from build123d import *

# Parameters (mm, degrees)
CROQUIS1_R              = 1.5
SALIENTE_EXTRUIR1_DEPTH = 3


with BuildPart() as part:
    # Croquis1 → Saliente-Extruir1 (new body)
    with BuildSketch(Plane(origin=(0, 0, 0), x_dir=(1, 0, 0), z_dir=(0, 1, 0))):
        with BuildLine():
            Line((-27.161614769, -3.105), (-9.331998714, -3.105))
            ThreePointArc((-9.331998714, -3.105), (2.40938914, -9.535306444), (9.686839463, 1.700695802))
            Line((9.686839463, 1.700695802), (11.574510255, 2.02597122))
            ThreePointArc((11.574510255, 2.02597122), (13.368530359, 5.198598559), (9.902464329, 6.325744796))
            Line((9.902464329, 6.325744796), (8.227399936, 5.249463408))
            ThreePointArc((8.227399936, 5.249463408), (7.196926129, 5.010869422), (6.248965214, 5.480095872))
            ThreePointArc((6.248965214, 5.480095872), (5.907504818, 6.481199341), (6.278579258, 7.471707855))
            Line((6.278579258, 7.471707855), (7.564320065, 8.991935775))
            ThreePointArc((7.564320065, 8.991935775), (6.899293653, 12.575483213), (3.519617395, 11.210983026))
            Line((3.519617395, 11.210983026), (2.928263966, 9.309793011))
            ThreePointArc((2.928263966, 9.309793011), (2.29224049, 8.464643619), (1.264447351, 8.214754404))
            ThreePointArc((1.264447351, 8.214754404), (0.359376606, 8.762157641), (0.006949519, 9.759453236))
            Line((0.006949519, 9.759453236), (0.014700448, 11.750473647))
            ThreePointArc((0.014700448, 11.750473647), (-2.798199231, 14.068159511), (-4.510097634, 10.850477702))
            Line((-4.510097634, 10.850477702), (-3.741039257, 9.013966998))
            ThreePointArc((-3.741039257, 9.013966998), (-3.685009949, 7.957716993), (-4.31171948, 7.105638053))
            ThreePointArc((-4.31171948, 7.105638053), (-5.356907913, 6.943205), (-6.267931977, 7.480641985))
            Line((-6.267931977, 7.480641985), (-7.541797671, 9.010834307))
            ThreePointArc((-7.541797671, 9.010834307), (-11.186383596, 8.978187623), (-10.429487856, 5.412913271))
            Line((-10.429487856, 5.412913271), (-8.659868635, 4.500405648))
            ThreePointArc((-8.659868635, 4.500405648), (-8.038781185, 3.922072963), (-7.809412295, 3.105))
            Line((-7.809412295, 3.105), (-27.161614769, 3.105))
            ThreePointArc((-27.161614769, 3.105), (-30.266614769, 0), (-27.161614769, -3.105))
        make_face()
        with Locations(Location((0, 0, 0), (0, 0, 270))):
            Circle(CROQUIS1_R, mode=Mode.SUBTRACT)
        with Locations(Location((-27.161614769, 0, 0), (0, 0, 270))):
            Circle(CROQUIS1_R, mode=Mode.SUBTRACT)
    extrude(amount=SALIENTE_EXTRUIR1_DEPTH)


solid = part.part
CAD build for the part. Positions are in the model's coordinates, mm. A direction names the side the tool comes from. Give positions to 0.01 mm unless a question says otherwise; leave off trailing zeros. Order: outer loops, then holes, each group sorted by start corner. A loop starts at its lowest first (then second) coordinate and runs counter-clockwise, first axis right, second up. Notation, with made-up numbers: (29, 3) - (40, 3) arc R19 cw to (40, 21) - close; hole circle Ø3 at (-8.75, 22). An arc over 180 degrees is marked (long way). Answer in a Markdown table with one row per item.
1. Flat gauge pins, fed straight in: pin 1 (1 mm diameter, centred on y = 0.5, z = 4.5, fed in from +X); pin 2 (0.9 mm diameter, centred on x = -22.5, y = 1.5, fed in from +Z) (3 decimals). Where does each tip first touch, or does it go through?
Data:
| item | result |
|---|---|
| pin 1 | stops at x = 8.98 |
| pin 2 | stops at z = 3.105 |
2. Saw through at D-D, the plane z = 5.5. Give the cut face in (x, y).
Data:
| item | result |
|---|---|
| outline | (-8.15, 0) - (8.15, 0) - (8.15, 3) - (-8.15, 3) - close |
3. Tool access for faces 1 (the flat face through (-17, 1, -3.105)), 2 (the flat face through (-4.131, 1.479, -9.945)), 3 (the flat face through (-6.9, 1.48, -8.24)), 4 (the flat face through (6.91, 1.48, -8.22)): list every direction of +Z, -Z, +X, -X, +Y, -Y with a clear straight run to the whole face (end or side of a thin tool).
Data:
| item | result |
|---|---|
| face 1 | -X, +Y, -Y |
| face 2 | +Y, -Y |
| face 3 | -Z, +Y, -Y |
| face 4 | +X, +Y, -Y |
4. Pull direction Z, two halves, no side cores. Call faces 5 (the flat face through (3.228, 1.479, -10.274)), 6 (the cylindrical face through (-8.045, 1.479, -3.932)), 7 (the flat face through (-4, 3, -2)), 8 (the cylindrical face through (-30.266, 1.479, -0.068)): pulls with the +Z half, pulls with the -Z half, needs draft (parallel to the pull), parting line crosses it, or undercut.
Data:
| item | result |
|---|---|
| face 5 | pulls with the -Z half |
| face 6 | undercut |
| face 7 | needs draft |
| face 8 | parting line crosses it |
5. Saw through at C-C, the plane x = -0.5. Give the cut face in (y, z), plus the area to 3 significant figures.
Data:
| item | result |
|---|---|
| outline | (0, -13.23) - (3, -13.23) - (3, -1.41) - (0, -1.41) - close; (0, 1.41) - (3, 1.41) - (3, 9.82) - (0, 9.82) - close |
| area | 60.7 mm² |
6. Probe probe 1 along X at (y, z) = (2.35, 0) (3 decimals); probe 2 along X at (y, z) = (1.9, -0.5); probe 3 along Z at (x, y) = (-9, 2.3) (3 decimals). List the from-to ranges inside material, lowest first. Write a range as [from, to].
Data:
| item | result |
|---|---|
| probe 1 | x = [-30.267, -28.662], [-25.662, -1.5], [1.5, 9.835] |
| probe 2 | x = [-30.23, -28.58], [-25.75, -1.41], [1.41, 9.82] |
| probe 3 | z = [-9.832, -4.676], [-3.105, 3.966] |
7. Saw through at B-B, the plane y = 2.35. Give the cut face in (x, z) (1 decimal), plus the area to 3 significant figures.
Data:
| item | result |
|---|---|
| outline | (-27.2, -3.1) - (-7.8, -3.1) arc R1.6 cw to (-8.7, -4.5) - (-10.4, -5.4) arc R2.4 ccw (long way) to (-7.5, -9) - (-6.3, -7.5) arc R1.6 cw to (-4.3, -7.1) arc R1.6 cw to (-3.7, -9) - (-4.5, -10.9) arc R2.4 ccw (long way) to (0, -11.8) - (0, -9.8) arc R1.6 cw to (1.3, -8.2) arc R1.6 cw to (2.9, -9.3) - (3.5, -11.2) arc R2.4 ccw (long way) to (7.6, -9) - (6.3, -7.5) arc R1.6 cw to (6.2, -5.5) arc R1.6 cw to (8.2, -5.2) - (9.9, -6.3) arc R2.4 ccw (long way) to (11.6, -2) - (9.7, -1.7) arc R9.8 ccw to (-9.3, 3.1) - (-27.2, 3.1) arc R3.1 ccw to start; hole circle Ø3 at (-27.2, 0); hole circle Ø3 at (0, 0) |
| area | 475 mm² |
8. Saw through at A-A, the plane z = 0. Give the cut face in (x, y) (3 decimals), plus the area to 3 significant figures.
Data:
| item | result |
|---|---|
| outline | (-30.267, 0) - (-28.662, 0) - (-28.662, 3) - (-30.267, 3) - close; (-25.662, 0) - (-1.5, 0) - (-1.5, 3) - (-25.662, 3) - close; (1.5, 0) - (9.835, 0) - (9.835, 3) - (1.5, 3) - close |
| area | 102 mm² |
